Job drawing, mm, ordinate dimensions from the low corner. One solid piece. A direction names the side the tool comes from. Give positions to 0.01 mm unless a question says otherwise; leave off trailing zeros. Order: outer loops, then holes, each group sorted by start corner. A loop starts at its lowest first (then second) coordinate and runs counter-clockwise, first axis right, second up.
1. Slice it at B-B on y = 56. List the corners of the cut face in (x, z).
2. Slice it at C-C on x = 20. List the corners of the cut face in (y, z).
3. Probe line 1 (Y direction, x = 32, z = 10.05); line 2 (Y direction, x = 32, z = 4.5); line 3 (X direction, y = 23.5, z = 7). List the from-to ranges inside material, lowest first.
4. Mould opens along X. For the marked faces 1, 2 and 3 say: +X half, -X half, draft (parallel to the pull), parting line (faces both ways), or undercut.
5. Drop flat-ended pins along their axis: pin 1 Ø23.5 at (x, y) = (32, 56) entering from +Z; pin 2 Ø4 at (x, z) = (59, 9.5) entering from -Y (3 decimals). Give the stop position or say it passes through.
6. Which spindle directions (+Z, -Z, +X, -X, +Y, -Y) get a long thin tool onto all of the face, cutting with end or side? Do the marked faces 4 and 5. Say none if no direction does.
7. Slice it at A-A on x = 32. List the corners of the cut face in (y, z), and give its area (3 significant figures).
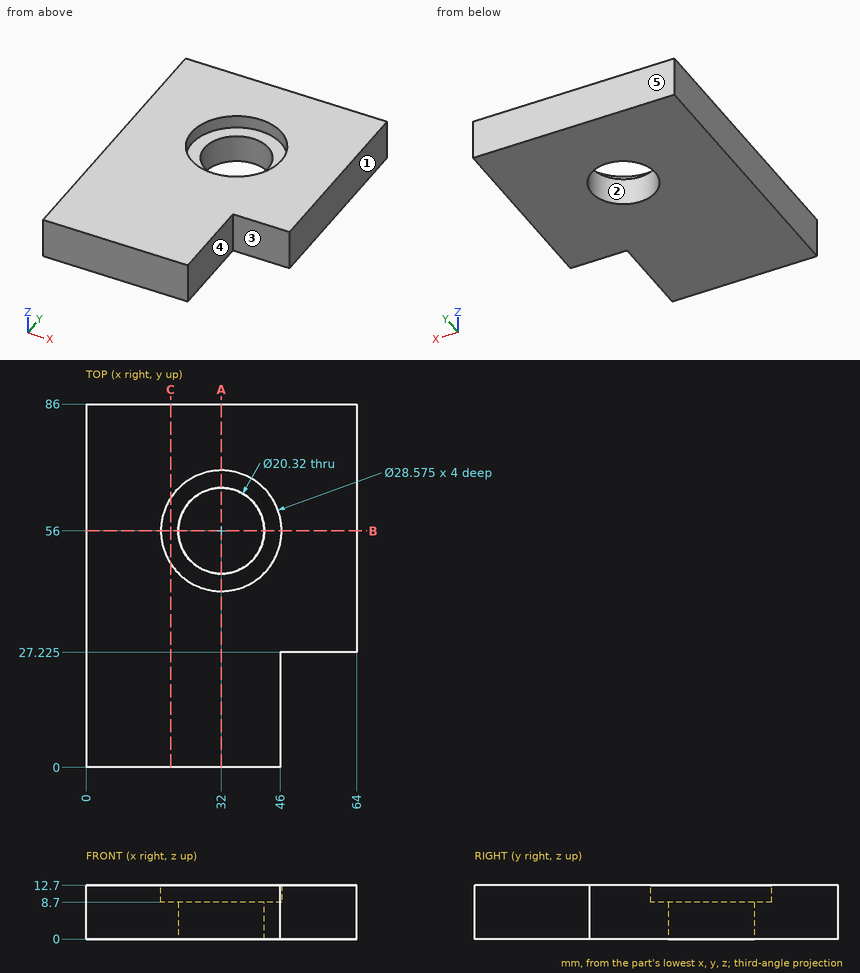
Data:
1. outline: (0, 0) - (21.84, 0) - (21.84, 8.7) - (17.71, 8.7) - (17.71, 12.7) - (0, 12.7) - close; (42.16, 0) - (64, 0) - (64, 12.7) - (46.29, 12.7) - (46.29, 8.7) - (42.16, 8.7) - close
2. outline: (0, 0) - (86, 0) - (86, 12.7) - (63.75, 12.7) - (63.75, 8.7) - (48.25, 8.7) - (48.25, 12.7) - (0, 12.7) - close
3. line 1: y = 0 to 41.71, 70.29 to 86
3. line 2: y = 0 to 45.84, 66.16 to 86
3. line 3: x = 0 to 46
4. face 1: +X half
4. face 2: undercut
4. face 3: draft
5. pin 1: stops at z = 8.7
5. pin 2: stops at y = 27.225
6. face 4: +Z, -Z, +X, -Y
6. face 5: +Z, -Z, +X, -X, +Y
7. outline: (0, 0) - (45.84, 0) - (45.84, 8.7) - (41.71, 8.7) - (41.71, 12.7) - (0, 12.7) - close; (66.16, 0) - (86, 0) - (86, 12.7) - (70.29, 12.7) - (70.29, 8.7) - (66.16, 8.7) - close
7. area: 801 mm2
